Geometry: final body of the model. Coordinates: model frame, mm. A direction names the side the tool comes from. Give positions to 0.01 mm unless a question says otherwise; leave off trailing zeros. Loops run counter-clockwise (first coordinate to the right, second up) from the corner with the lowest first, then second, coordinate; pieces in that order, holes last. Notation, with made-up numbers: (38.5, 36.25) - (57.5, 36.25) arc R24 ccw to (57.5, 64.25) - close; hole circle Ø5 at (1, 47.5). An arc over 180 degrees is marked (long way). Answer in a Markdown table with one row per item.
from build123d import *

# Parameters (mm, degrees)
F1_DEPTH = 20
F3_D     = 10
F3_DEPTH = 45
F3_TIP   = 3.0043030951
F4_W     = 15
F4_H     = 20
F5_DEPTH = 2
F6_DEPTH = 26.501
F7_SIZE  = 1.5


with BuildPart() as f1:
    # F0 (on Front) → F1 (new body)
    with BuildSketch(Plane.XZ):
        with BuildLine():
            Line((7.5, 35), (0, 35))
            Line((0, 35), (-7.5, 35))
            Line((-7.5, 35), (-7.5, 0))
            Line((-7.5, 0), (-5.5, 0))
            Line((-5.5, 0), (-5.5, 31))
            ThreePointArc((-5.5, 31), (-4.9142135624, 32.4142135624), (-3.5, 33))
            Line((-3.5, 33), (0, 33))
            Line((0, 33), (3.5, 33))
            ThreePointArc((3.5, 33), (4.9142135624, 32.4142135624), (5.5, 31))
            Line((5.5, 31), (5.5, 0))
            Line((5.5, 0), (7.5, 0))
            Line((7.5, 0), (7.5, 35))
        make_face()
    extrude(amount=F1_DEPTH)

    # F3
    with Locations(Plane(origin=(-7.5, 0, 0), x_dir=(0, -1, 0), z_dir=(-1, 0, 0))):
        with Locations((10, 10)):
            Hole(F3_D / 2, depth=F3_DEPTH)
            with Locations((0, 0, -(F3_DEPTH + F3_TIP / 2))):  # 118° drill point
                Cone(0, F3_D / 2, F3_TIP, mode=Mode.SUBTRACT)

    # F4 (on face) → F5 (join)
    with BuildSketch(Plane.XY.offset(35)):
        with BuildLine():
            Line((5, -33), (15.5, -33))
            ThreePointArc((15.5, -33), (16.9142135624, -32.4142135624), (17.5, -31))
            Line((17.5, -31), (17.5, -15))
            Line((17.5, -15), (17.5, -5))
            Line((17.5, -5), (17.5, 11))
            ThreePointArc((17.5, 11), (16.9142135624, 12.4142135624), (15.5, 13))
            Line((15.5, 13), (5, 13))
            Line((5, 13), (0, 13))
            Line((0, 13), (-5, 13))
            Line((-5, 13), (-15.5, 13))
            ThreePointArc((-15.5, 13), (-16.9142135624, 12.4142135624), (-17.5, 11))
            Line((-17.5, 11), (-17.5, -5))
            Line((-17.5, -5), (-17.5, -10))
            Line((-17.5, -10), (-17.5, -15))
            Line((-17.5, -15), (-17.5, -31))
            ThreePointArc((-17.5, -31), (-16.9142135624, -32.4142135624), (-15.5, -33))
            Line((-15.5, -33), (-5, -33))
            Line((-5, -33), (5, -33))
        make_face()
        with Locations((0, -10)):
            Rectangle(F4_W, F4_H, mode=Mode.SUBTRACT)
        Polygon((5, -34.5), (5, -33), (-5, -33), (-5, -34.5), (0, -34.5), align=None)
        Polygon((17.5, -5), (17.5, -15), (19, -15), (19, -10), (19, -5), align=None)
        Polygon((-19, -15), (-17.5, -15), (-17.5, -10), (-17.5, -5), (-19, -5), (-19, -10), align=None)
        Polygon((0, 13), (5, 13), (5, 14.5), (0, 14.5), (-5, 14.5), (-5, 13), align=None)
        with Locations((0, -10)):
            Rectangle(F4_W, F4_H)
    extrude(amount=F5_DEPTH)

    # F2 (on face) → F6 (cut, through all)
    with BuildSketch(Plane(origin=(-7.5, 0, 0), x_dir=(0, -1, 0), z_dir=(-1, 0, 0))):
        with BuildLine():
            Line((20, 0), (20, 5))
            ThreePointArc((20, 5), (18.5355339059, 1.4644660941), (15, 0))
            Line((15, 0), (20, 0))
        make_face()
        with BuildLine():
            ThreePointArc((5, 0), (1.4644660941, 1.4644660941), (0, 5))
            Line((0, 5), (0, 0))
            Line((0, 0), (5, 0))
        make_face()
    extrude(amount=-F6_DEPTH, mode=Mode.SUBTRACT)

    # F7
    f7_edges = [f1.edges().sort_by_distance(p)[0] for p in [
        (-19, -10, 35),
        (0, 14.5, 35),
        (19, -10, 35),
        (0, -34.5, 35),
    ]]
    chamfer(f7_edges, length=F7_SIZE)


solid = f1.part
Q1. Cut plane B-B (y = -10). Output: boundary loops of the cut face in (x, z), and give its area (3 significant figures).
Check values:
| item | result |
|---|---|
| outline | (-19, 36.5) - (-17.5, 35) - (-7.5, 35) - (-7.5, 15) - (-5.5, 15) - (-5.5, 31) arc R2 cw to (-3.5, 33) - (3.5, 33) arc R2 cw to (5.5, 31) - (5.5, 15) - (7.5, 15) - (7.5, 35) - (17.5, 35) - (19, 36.5) - (19, 37) - (-19, 37) - close; (-7.5, 0) - (-5.5, 0) - (-5.5, 5) - (-7.5, 5) - close; (5.5, 0) - (7.5, 0) - (7.5, 5) - (5.5, 5) - close |
| area | 197 mm² |
Q2. Cut plane D-D (x = 2). Output: boundary loops of the cut face in (y, z).
Check values:
| item | result |
|---|---|
| outline | (-34.5, 36.5) - (-33, 35) - (-20, 35) - (-20, 33) - (0, 33) - (0, 35) - (13, 35) - (14.5, 36.5) - (14.5, 37) - (-34.5, 37) - close |
Q3. Cut plane A-A (z = 7). Output: boundary loops of the cut face in (x, y), and give its area (3 significant figures).
Check values:
| item | result |
|---|---|
| outline | (-7.5, -20) - (-5.5, -20) - (-5.5, -14) - (-7.5, -14) - close; (-7.5, -6) - (-5.5, -6) - (-5.5, 0) - (-7.5, 0) - close; (5.5, -20) - (7.5, -20) - (7.5, -14) - (5.5, -14) - close; (5.5, -6) - (7.5, -6) - (7.5, 0) - (5.5, 0) - close |
| area | 48.0 mm² |
Q4. Draft query along X for faces 6 (the flat face through (18, -5, 36)), 7 (the flat face through (-5.5, -9.9, 15.3)), 8 (the flat face through (-17.5, 3, 36)). Return one class per face: pulls with the +X half, pulls with the -X half, needs draft (parallel to the pull), parting line crosses it, or undercut.
Check values:
| item | result |
|---|---|
| face 6 | needs draft |
| face 7 | undercut |
| face 8 | pulls with the -X half |
Q5. First-contact query: pin 1 (1 mm diameter, centred on y = -19, z = 32.5, fed in from +X); pin 2 (1 mm diameter, centred on y = 5.5, z = 36, fed in from -X); pin 3 (1 mm diameter, centred on y = -25, z = 36, fed in from +X). Flat tips, straight axial feed; report the tip coordinate or a pass-through.
Check values:
| item | result |
|---|---|
| pin 1 | x = 7.5 |
| pin 2 | x = -17.5 |
| pin 3 | x = 17.5 |
Q6. Reachability of faces 1 (the flat face through (5, -33.6, 36.2)), 2 (the flat face through (5.5, -10, 16)), 3 (the flat face through (6, 0, 22)), 4 (the flat face through (5, 13.6, 36.2)), 5 (the flat face through (-10, 13, 36)) from +Z, -Z, +X, -X, +Y, -Y: full face, straight path, thin tool, end or side. Return the list, or none.
Check values:
| item | result |
|---|---|
| face 1 | +Z, -Z, +X, -Y |
| face 2 | -Z, +Y, -Y |
| face 3 | -Z, +X, -X, +Y |
| face 4 | +Z, -Z, +X, +Y |
| face 5 | +Z, -Z, -X, +Y |
Q7. Material intervals for line 1 along Z through (x, y) = (6, -10); line 2 along X through (y, z) = (-7.5, 21); line 3 along Z through (x, y) = (-12, -1), sorted ascending.
Check values:
| item | result |
|---|---|
| line 1 | 0 to 5, 15 to 37 |
| line 2 | -7.5 to -5.5, 5.5 to 7.5 |
| line 3 | 35 to 37 |
Q8. Cut plane C-C (z = 22.5). Output: boundary loops of the cut face in (x, y).
Check values:
| item | result |
|---|---|
| outline | (-7.5, -20) - (-5.5, -20) - (-5.5, 0) - (-7.5, 0) - close; (5.5, -20) - (7.5, -20) - (7.5, 0) - (5.5, 0) - close |
